Autodesk Inventor part; units mm, degrees
ref_plane "YZ Plane" through (0, 0, 0) normal (1, 0, 0) x (0, 1, 0)
ref_plane "XZ Plane" through (0, 0, 0) normal (0, 1, 0) x (-1, 0, 0)
ref_plane "XY Plane" through (0, 0, 0) normal (0, 0, 1) x (1, 0, 0)
sketch "Sketch1" plane through (0, 0, 0) normal (0, 1, 0) x (-1, 0, 0)
  circle A0 centre (0, 0) radius 4.025
  line L0 (0, 0) -> (36.11, 0) construction
  line L1 (0, -10) -> (36.11, -10)
  line L2 (36.11, 10) -> (0, 10)
  arc A1 (0, 10) -> (0, -10) centre (0, 0) ccw
  line L3 (36.11, 10) -> (36.11, -10)
  point P0 (18.055, 0)
  dimension "d0" = 8.05
  dimension "d1" = 36.11
extrude "Extrusion1" add sketch "Sketch1" along normal blind 8
sketch "Sketch2" plane through (-36.11, 0, 10) normal (0, 0, 1) x (1, 0, 0)
  line L0 (0, 0) -> (0, 8)
  line L1 (36.11, 0) -> (0, 0)
  line L2 (0, 8) -> (8, 8)
  line L3 (8, 8) -> (8, 0)
  line L4 (8, 0) -> (0, 0)
  line L5 (0, 0) -> (0, 8)
  dimension "d5" = 8
extrude "Extrusion2" add sketch "Sketch2" along normal blind 23.06
sketch "Sketch3" plane through (-28.11, 0, 10) normal (1, 0, 0) x (0, 0, -1)
  circle A0 centre (-18.06, 4) radius 2.2
  line L0 (-23.06, 0) -> (-23.06, 8)
  point P0 (10, 0)
  point P1 (-23.06, 4)
  dimension "d8" = 4.4
  dimension "d9" = 5
extrude "Extrusion3" cut sketch "Sketch3" against normal blind 23.06
sketch "Sketch4" plane through (0, 0, -10) normal (0, 0, -1) x (-1, 0, 0)
  line L0 (36.11, 0) -> (36.11, 8)
  line L1 (28.11, 0) -> (28.11, 8)
  line L2 (36.11, 8) -> (28.11, 8)
  line L3 (28.11, 8) -> (28.11, 0)
  line L4 (28.11, 0) -> (36.11, 0)
  line L5 (36.11, 0) -> (36.11, 8)
  point P0 (0, 0)
extrude "Extrusion4" add sketch "Sketch4" along normal blind 14.94
sketch "Sketch6" plane through (-36.11, 0, 33.06) normal (-1, 0, 0) x (0, 0, 1)
  circle A0 centre (-21, 4) radius 1.95
  circle A1 centre (-5, 4) radius 2.2
  circle A2 centre (-37, 4) radius 1.95
  circle A3 centre (-53, 4) radius 2.2
  point P0 (-33.06, 0)
  dimension "d18" = 3.9
  dimension "d19" = 16
  dimension "d20" = 3.9
  dimension "d21" = 16
  dimension "d22" = 4.4
  dimension "d23" = 16
extrude "Extrusion6" add sketch "Sketch6" along normal blind 2 contours A0 | A2
extrude "Extrusion7" cut sketch "Sketch6" against normal blind 13 contours A3
sketch "Sketch7" plane through (0, 8, 0) normal (0, 1, 0) x (1, 0, 0)
  point P0 (0, 0)
sketch "Sketch8" plane through (0, 8, 0) normal (0, 1, 0) x (1, 0, 0)
  line L0 (-28.11, -10) -> (-28.11, -33.06) construction
  line L1 (-28.11, -28.0914) -> (-28.11, -18.1514)
  line L2 (-28.11, -18.1514) -> (-19.9586, -10)
  line L3 (-28.11, -10) -> (0, -10)
  line L4 (-28.11, -18.1514) -> (-16.5822, -18.1514) construction
  line L5 (-19.9586, -10) -> (-28.11, -10)
  line L6 (-28.11, -10) -> (-28.11, -18.1514)
  point P0 (0, 0)
  dimension "d31" = 9.94
  dimension "d32" = 45
extrude "Extrusion8" add sketch "Sketch8" against normal blind 8
chamfer "Chamfer1" distance 4 angle 45 1 edges at (-28.11, 4, -10)
properties part number "Launcher_support"
Model file for the job. Use its own axes, mm. A direction names the side the tool comes from. Give positions to 0.01 mm unless a question says otherwise; leave off trailing zeros. Order: outer loops, then holes, each group sorted by start corner. A loop starts at its lowest first (then second) coordinate and runs counter-clockwise, first axis right, second up. Notation, with made-up numbers: (-21, 78.5) - (5, 78.5) arc R25 ccw to (5, 94.5) - close; hole circle Ø9 at (-12, -14.5). An arc over 180 degrees is marked (long way). Write item = value, one per line. Start each with the question number.
1. Which spindle directions (+Z, -Z, +X, -X, +Y, -Y) get a long thin tool onto all of the face, cutting with end or side? Do faces 1 (the flat face through (-19, 8, 4)), 2 (the flat face through (-28.11, 6, -18)), 3 (the cylindrical face through (-37.096, 5.187, -5.487)), 4 (the flat face through (-32, 4, -24.94)), 5 (the flat face through (-10, 4, 10)). Say none if no direction does.
2. Cut at D-D, the plane x = -30. List the corners of the cut face in (y, z).
3. Drop flat-ended pins along their axis: P1, Ø2.5, axis at y = 2.5, z = 4.5, coming from the -X side; P2, Ø2.5, axis at x = -17.5, y = 3.5, coming from the -Z side; P3, Ø3.5, axis at y = 4, z = -19.94, coming from the +X side; P4, Ø2.5, axis at x = -10.5, y = 2.5, coming from the +Z side. Give the stop position or say it passes through.
4. Cut at B-B, the plane y = 4. List the corners of the cut face in (x, z) (3 decimals).
5. Two-plate mould, pull along Z, no slides. Class faces 6 (the flat face through (-38.11, 4, -4)), 7 (the cylindrical face through (-32.054, 4.097, 30.258)), 8 (the flat face through (-12, 4, -10)): pulls with the +Z half, pulls with the -Z half, needs draft (parallel to the pull), parting line crosses it, or undercut.
6. Cut at A-A, the plane z = 0. List the corners of the cut face in (x, y) (3 decimals).
7. Probe line 1 along Z through (x, y) = (0, 4.5) (3 decimals); line 2 along Y through (x, z) = (-30.25, -19.94); line 3 along Z through (x, y) = (-5, 1.75). List the from-to ranges inside material, lowest first.
8. Cut at C-C, the plane x = 1. List the corners of the cut face in (y, z).
Taken from the geometry:
q1.face_1 = +Z, -Z, +X, -X, +Y
q1.face_2 = -Z, +X, +Y, -Y
q1.face_3 = -X
q1.face_4 = -Z, +X, -X, +Y, -Y
q1.face_5 = +Z, +X, +Y, -Y
q2.outline = (0, -24.94) - (8, -24.94) - (8, 33.06) - (0, 33.06) - close; hole circle Ø4.4 at (4, -19.94); hole circle Ø4.4 at (4, 28.06)
q3.P1 = -36.11
q3.P2 = -10
q3.P3 = through
q3.P4 = 10
q4.outline = (-38.11, -5.89) - (-36.11, -5.89) - (-36.11, -17.74) - (-28.11, -17.74) - (-28.11, -14) - (-24.11, -10) - (0, -10) arc R10 ccw to (0, 10) - (-19.959, 10) - (-28.11, 18.151) - (-28.11, 25.86) - (-36.11, 25.86) - (-36.11, 14.01) - (-38.11, 14.01) - (-38.11, 10.11) - (-36.11, 10.11) - (-36.11, -1.99) - (-38.11, -1.99) - close; (-36.11, -24.94) - (-28.11, -24.94) - (-28.11, -22.14) - (-36.11, -22.14) - close; (-36.11, 30.26) - (-28.11, 30.26) - (-28.11, 33.06) - (-36.11, 33.06) - close; hole circle Ø8.05 at (0, 0)
q5.face_6 = needs draft
q5.face_7 = undercut
q5.face_8 = pulls with the -Z half
q6.outline = (-36.11, 0) - (-4.025, 0) - (-4.025, 8) - (-36.11, 8) - close; (4.025, 0) - (10, 0) - (10, 8) - (4.025, 8) - close
q7.line_1 = -10 to -4.025, 4.025 to 10
q7.line_2 = 0 to 1.8, 6.2 to 8
q7.line_3 = -10 to 10
q8.outline = (0, -9.95) - (8, -9.95) - (8, -3.9) - (0, -3.9) - close; (0, 3.9) - (8, 3.9) - (8, 9.95) - (0, 9.95) - close
